Input: part model. Units: mm. Frame: model coordinates. Face numbers are marked on the shaded views. A direction names the side the tool comes from. Round coordinates to 2 decimals unless told otherwise and drop trailing zeros. Loops run counter-clockwise (first coordinate to the right, second up) from the corner with the lowest first, then second, coordinate; pieces in that order, holes last. Notation, with made-up numbers: M 30,-39.75 L 44,-39.75 A24 cw 44,-15.75 Z; hole C -6.75,0 d4. An arc over 180 degrees is marked long. Use one line per item in the form item = value. Start each with the question number.
Q1. Section query B-B, the plane y = 24.5. Output: boundary loops of the cut face in (x, z), and give its area (3 significant figures).
Q2. Section query A-A, the plane z = -35. Output: boundary loops of the cut face in (x, y), and give its area (3 significant figures).
Q3. First-contact query: P1, Ø2, axis at x = 9, y = 56.5, coming from the +Z side; P2, Ø2, axis at x = 5.5, y = 28, coming from the +Z side. Flat tips, straight axial feed; report the tip coordinate or a pass-through.
Q4. Ray query, line 1 along X through (y, z) = (42, -8); line 2 along X through (y, z) = (34, 1.5); line 3 along Z through (x, y) = (14, 43.5). Return the intervals inside material, ascending.
Q5. Section query C-C, the plane x = 10.5. Output: boundary loops of the cut face in (y, z).
Q6. Mould query, pull axis Z, two halves, no side actions, for the marked faces 3, 4 and 5. Classes: pulls with the +Z half, pulls with the -Z half, needs draft (parallel to the pull), parting line crosses it, or undercut.
Q7. Section query D-D, the plane y = 44.5. Output: boundary loops of the cut face in (x, z), and give its area (3 significant figures).
Q8. Access query for the marked faces 1 and 2. Directions: +Z, -Z, +X, -X, +Y, -Y. A direction counts if a zero-diameter tool reaches every point of the face in a straight line with its end or side. Return the directions, or none.
```python
from build123d import *

# Parameters (mm, degrees)
F1_DEPTH = 63.5
F3_DEPTH = 25.4


with BuildPart() as f1:
    # F0 (on Front) → F1 (new body)
    with BuildSketch(Plane.XZ):
        Polygon((-63.103128, 16.393103), (-63.103128, -47.106897), (25.796872, -47.106897), (-25.003128, 16.393103), align=None)
    extrude(amount=-F1_DEPTH)

    # F2 (on face) → F3 (join)
    with BuildSketch(Plane(origin=(-7.249174, 0, -5.799339), x_dir=(0, 1, 0), z_dir=(0.780869, 0, 0.624695))):
        Polygon((55.396065, -24.504127), (37.371274, -14.751914), (41.925259, -38.956322), align=None)
    extrude(amount=F3_DEPTH)


solid = f1.part
```
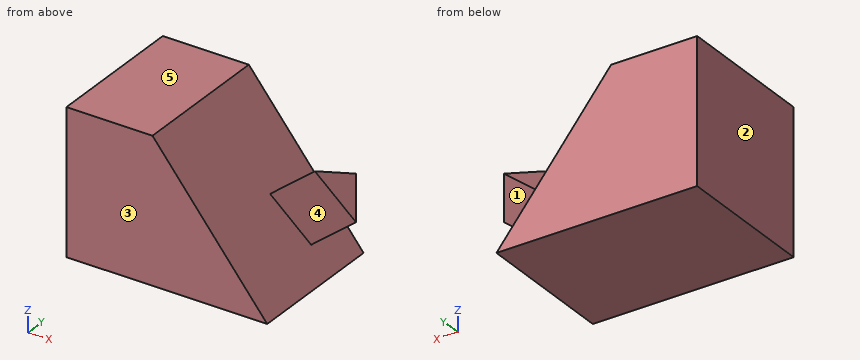
Results found:
q1.outline = M -63.1,-47.11 L 25.8,-47.11 L -25,16.39 L -63.1,16.39 Z
q1.area = 4,030 mm²
q2.outline = M -63.1,0 L 16.11,0 L 16.11,41.63 L 18.61,41.93 L 16.11,43.38 L 16.11,63.5 L -63.1,63.5 Z
q2.area = 5,030 mm²
q3.P1 = -24.86
q3.P2 = -20.49
q4.line_1 = -63.1 to -5.49, 17.62 to 27.04
q4.line_2 = -63.1 to -13.09
q4.line_3 = -47.11 to -11.94
q5.outline = M 0,-47.11 L 63.5,-47.11 L 63.5,-27.99 L 51.75,-27.99 L 55.4,-22.98 L 37.37,-10.49 L 39.94,-27.99 L 0,-27.99 Z
q6.face_3 = needs draft
q6.face_4 = undercut
q6.face_5 = pulls with the +Z half
q7.outline = M -63.1,-47.11 L 25.8,-47.11 L 15.36,-34.06 L 35.2,-18.19 L 24.21,-4.46 L 4.38,-20.33 L -25,16.39 L -63.1,16.39 Z
q7.area = 4,480 mm²
q8.face_1 = +X, +Y
q8.face_2 = +Z, -Z, -X, +Y, -Y
